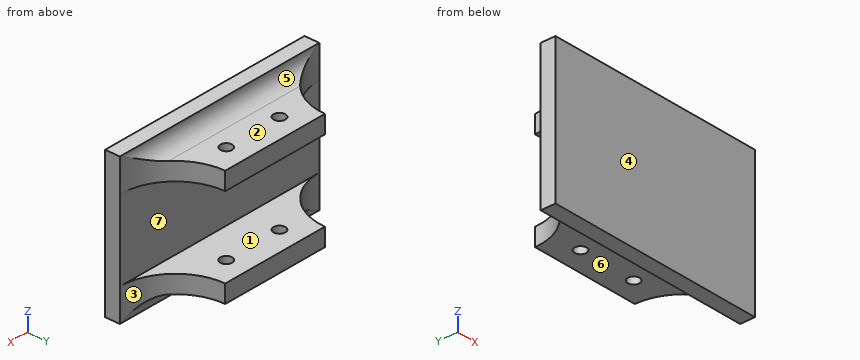
Autodesk Inventor part; units mm, degrees
ref_plane "YZ Plane" through (0, 0, 0) normal (1, 0, 0) x (0, 1, 0)
ref_plane "XZ Plane" through (0, 0, 0) normal (0, 1, 0) x (-1, 0, 0)
ref_plane "XY Plane" through (0, 0, 0) normal (0, 0, 1) x (1, 0, 0)
sketch "Sketch1" plane through (0, 0, 0) normal (0, 1, 0) x (-1, 0, 0)
  line L0 (75, 49) -> (75, -49)
  line L1 (75, -49) -> (-75, -49)
  line L2 (-75, -49) -> (-75, 49)
  line L3 (-75, 49) -> (75, 49)
  point P0 (0, 0)
  dimension "d0" = 98
  dimension "d1" = 150
  dimension "d2" = 75
  dimension "d3" = 49
extrude "Extrusion1" add sketch "Sketch1" along normal blind 10
sketch "Sketch2" plane through (0, 10, 0) normal (0, 1, 0) x (1, 0, 0)
  line L0 (-37.5, -39) -> (-37.5, -27)
  line L1 (-37.5, -27) -> (37.5, -27)
  line L2 (37.5, -27) -> (37.5, -39)
  line L3 (37.5, -39) -> (-37.5, -39)
  line L4 (-75, -49) -> (75, -49)
  point P0 (0, 0)
  point P1 (-37.5, -33)
  dimension "d6" = 12
  dimension "d8" = 37.5
  dimension "d9" = 75
  dimension "d14" = 33
extrude "Extrusion2" add sketch "Sketch2" along normal blind 37.5
fillet "Face Fillet3" radius 10 1 edges at (0, 10, 39)
sketch "Sketch3" plane through (-37.5, 47.5, 39) normal (0, 0, 1) x (1, 0, 0)
  circle A0 centre (17.5, -15) radius 4
  circle A1 centre (57.5, -15) radius 4
  line L0 (-37.5, -47.5) -> (112.5, -47.5)
  line L1 (0, 0) -> (75, 0)
  point P0 (37.5, -47.5)
  point P1 (37.5, 0)
  dimension "d16" = 8
  dimension "d17" = 8
  dimension "d18" = 32.5
  dimension "d19" = 32.5
  dimension "d20" = 40
  dimension "d21" = 20
fillet "Face Fillet4" radius 37.5 1 edges at (37.5, 10, 33)
fillet "Face Fillet5" radius 37.5 1 edges at (-37.5, 10, 33)
extrude "Extrusion3" cut sketch "Sketch3" against normal blind 80
mirror "Mirror1" about plane through (0, 0, 0) normal (0, 0, 1) of "Extrusion2", "Face Fillet3", "Face Fillet4", "Face Fillet5", "Extrusion3"
thread "Thread5"
thread "Thread6"
thread "Thread7"
thread "Thread8"
properties part number "Base Macaco" material "Steel AISI 1050"
The listing builds one solid part. Answer for the finished solid, in the listing's coordinates (mm). Face numbers are marked on the shaded views. A direction names the side the tool comes from. Give positions to 0.01 mm unless a question says otherwise; leave off trailing zeros. Order: outer loops, then holes, each group sorted by start corner. A loop starts at its lowest first (then second) coordinate and runs counter-clockwise, first axis right, second up.
1) Find section A-A on z = 29.5. Give the number of separate pieces and of enclosed holes in the cut face, then the cut area to 3 significant figures.
Reported:
separate pieces: 1
enclosed holes: 2
area: 4,820 mm2
2) For the marked faces 1, 2 and 3, determine the directions among +Z, -Z, +X, -X, +Y, -Y from which every point of the face is accessible in a straight line to the end or side of a thin tool.
Reported:
face 1: +X, -X, +Y
face 2: +Z, +X, -X, +Y
face 3: +Z, -Z, +X, +Y
3) Given P1, Ø10.5, axis at x = 20, y = 32.5, coming from the +Z side; P2, Ø8.5, axis at x = 8.5, y = 28.5, coming from the -Z side; P3, Ø1.5, axis at x = -46.5, z = -32, coming from the +Y side, each flat-ended and moving along its own axis, determine where each tip first touches the part or whether it passes through.
Reported:
P1: stops at z = 39
P2: stops at z = -39
P3: stops at y = 24.03
4) Determine the mould class of the marked faces 4, 5, 6 and 7 for opening direction Z: pulls with the +Z half, pulls with the -Z half, needs draft (parallel to the pull), parting line crosses it, or undercut.
Reported:
face 4: needs draft
face 5: pulls with the +Z half
face 6: pulls with the -Z half
face 7: undercut
5) Find section D-D on y = 12. Write down the section's boundary in (x, z).
Reported:
outline: (-62.92, -43) - (62.92, -43) - (62.92, -27) - (-62.92, -27) - close; (-62.92, 27) - (62.92, 27) - (62.92, 43) - (-62.92, 43) - close
6) Consider line 1 along Y through (x, z) = (20, 30); line 2 along X through (y, z) = (32, 34); line 3 along Z through (x, y) = (-44.5, 22). Determine where each line is inside the solid, lowest interval first.
Reported:
line 1: y = 0 to 28.5, 36.5 to 47.5
line 2: x = -40.85 to -23.97, -16.03 to 16.03, 23.97 to 40.85
line 3: z = -39 to -27, 27 to 39
7) Find section C-C on y = 32.5. Write down the section's boundary in (x, z), then the cut area to 3 significant figures.
Reported:
outline: (-40.63, -39) - (-24, -39) - (-24, -27) - (-40.63, -27) - close; (-40.63, 27) - (-24, 27) - (-24, 39) - (-40.63, 39) - close; (-16, -39) - (16, -39) - (16, -27) - (-16, -27) - close; (-16, 27) - (16, 27) - (16, 39) - (-16, 39) - close; (24, -39) - (40.63, -39) - (40.63, -27) - (24, -27) - close; (24, 27) - (40.63, 27) - (40.63, 39) - (24, 39) - close
area: 1,570 mm2
